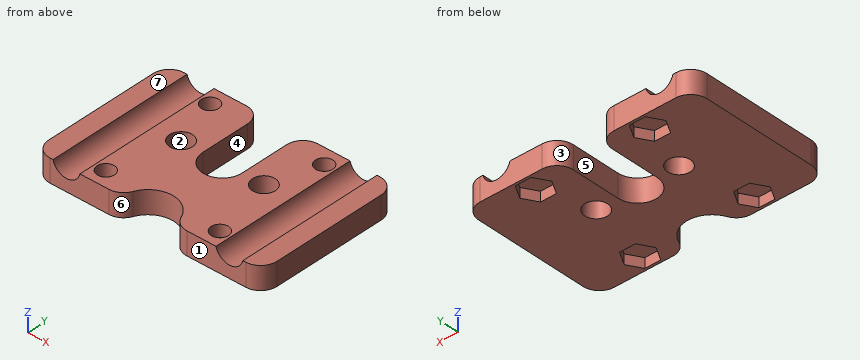
```python
from build123d import *

# Parameters (mm, degrees)
F0_R     = 3.5
F0_R_2   = 2.65
F1_DEPTH = 7
F2_DEPTH = 3
F3_R     = 4.25
F4_DEPTH = 45.001
F5_R     = 5
F7_R     = 2.65
F8_DEPTH = 0.25


with BuildPart() as f1:
    # F0 (on Top) → F1 (new body)
    with BuildSketch(Plane.XY):
        with BuildLine():
            Line((-6, 22.5), (-35, 22.5))
            Line((-35, 22.5), (-35, -22.5))
            Line((-35, -22.5), (-8, -22.5))
            ThreePointArc((-8, -22.5), (0, -14.5), (8, -22.5))
            Line((8, -22.5), (35, -22.5))
            Line((35, -22.5), (35, 22.5))
            Line((35, 22.5), (6, 22.5))
            Line((6, 22.5), (6, 2.5))
            ThreePointArc((6, 2.5), (0, -3.5), (-6, 2.5))
            Line((-6, 2.5), (-6, 22.5))
        make_face()
        Polygon((-22.4074772881, -17.5), (-19.9537386441, -13.25), (-15.0462613559, -13.25), (-12.5925227119, -17.5), (-15.0462613559, -21.75), (-19.9537386441, -21.75), align=None, mode=Mode.SUBTRACT)
        Polygon((12.5925227119, -17.5), (15.0462613559, -13.25), (19.9537386441, -13.25), (22.4074772881, -17.5), (19.9537386441, -21.75), (15.0462613559, -21.75), align=None, mode=Mode.SUBTRACT)
        with Locations((-12.7, 2.5)):
            Circle(F0_R, mode=Mode.SUBTRACT)
        Polygon((-12.5925227119, 17.5), (-15.0462613559, 13.25), (-19.9537386441, 13.25), (-22.4074772881, 17.5), (-19.9537386441, 21.75), (-15.0462613559, 21.75), align=None, mode=Mode.SUBTRACT)
        with Locations((12.7, 2.5)):
            Circle(F0_R, mode=Mode.SUBTRACT)
        Polygon((22.4074772881, 17.5), (19.9537386441, 13.25), (15.0462613559, 13.25), (12.5925227119, 17.5), (15.0462613559, 21.75), (19.9537386441, 21.75), align=None, mode=Mode.SUBTRACT)
        Polygon((-19.9537386441, 13.25), (-15.0462613559, 13.25), (-12.5925227119, 17.5), (-15.0462613559, 21.75), (-19.9537386441, 21.75), (-22.4074772881, 17.5), align=None)
        with Locations((-17.5, 17.5)):
            Circle(F0_R_2, mode=Mode.SUBTRACT)
        Polygon((-15.0462613559, -13.25), (-19.9537386441, -13.25), (-22.4074772881, -17.5), (-19.9537386441, -21.75), (-15.0462613559, -21.75), (-12.5925227119, -17.5), align=None)
        with Locations((-17.5, -17.5)):
            Circle(F0_R_2, mode=Mode.SUBTRACT)
        Polygon((19.9537386441, -13.25), (15.0462613559, -13.25), (12.5925227119, -17.5), (15.0462613559, -21.75), (19.9537386441, -21.75), (22.4074772881, -17.5), align=None)
        with Locations((17.5, -17.5)):
            Circle(F0_R_2, mode=Mode.SUBTRACT)
        Polygon((15.0462613559, 13.25), (19.9537386441, 13.25), (22.4074772881, 17.5), (19.9537386441, 21.75), (15.0462613559, 21.75), (12.5925227119, 17.5), align=None)
        with Locations((17.5, 17.5)):
            Circle(F0_R_2, mode=Mode.SUBTRACT)
    extrude(amount=F1_DEPTH)

    # F0 (on Top) → F2 (cut)
    with BuildSketch(Plane.XY):
        Polygon((19.9537386441, -13.25), (15.0462613559, -13.25), (12.5925227119, -17.5), (15.0462613559, -21.75), (19.9537386441, -21.75), (22.4074772881, -17.5), align=None)
        with Locations((17.5, -17.5)):
            Circle(F0_R_2, mode=Mode.SUBTRACT)
        Polygon((15.0462613559, 13.25), (19.9537386441, 13.25), (22.4074772881, 17.5), (19.9537386441, 21.75), (15.0462613559, 21.75), (12.5925227119, 17.5), align=None)
        with Locations((17.5, 17.5)):
            Circle(F0_R_2, mode=Mode.SUBTRACT)
        Polygon((-19.9537386441, 13.25), (-15.0462613559, 13.25), (-12.5925227119, 17.5), (-15.0462613559, 21.75), (-19.9537386441, 21.75), (-22.4074772881, 17.5), align=None)
        with Locations((-17.5, 17.5)):
            Circle(F0_R_2, mode=Mode.SUBTRACT)
        Polygon((-15.0462613559, -13.25), (-19.9537386441, -13.25), (-22.4074772881, -17.5), (-19.9537386441, -21.75), (-15.0462613559, -21.75), (-12.5925227119, -17.5), align=None)
        with Locations((-17.5, -17.5)):
            Circle(F0_R_2, mode=Mode.SUBTRACT)
    extrude(amount=F2_DEPTH, mode=Mode.SUBTRACT)

    # F3 (on face) → F4 (cut, through all)
    with BuildSketch(Plane(origin=(0, 22.5, 0), x_dir=(-1, 0, 0), z_dir=(0, 1, 0))):
        with Locations((-25, 8)):
            Circle(F3_R)
        with Locations((25, 8)):
            Circle(F3_R)
    extrude(amount=-F4_DEPTH, mode=Mode.SUBTRACT)

    # F5
    f5_edges = [f1.edges().sort_by_distance(p)[0] for p in [
        (35, 22.5, 3.5),
        (6, 22.5, 3.5),
        (-6, 22.5, 3.5),
        (-35, 22.5, 3.5),
        (-35, -22.5, 3.5),
        (35, -22.5, 3.5),
        (-8, -22.5, 3.5),
        (8, -22.5, 3.5),
    ]]
    fillet(f5_edges, radius=F5_R)

    # F7 (on offset) → F8 (join)
    with BuildSketch(Plane(origin=(0, 0, 3), x_dir=(1, 0, 0), z_dir=(0, 0, -1))):
        with Locations((17.5, -17.5)):
            Circle(F7_R)
        with Locations((17.5, 17.5)):
            Circle(F7_R)
        with Locations((-17.5, 17.5)):
            Circle(F7_R)
        with Locations((-17.5, -17.5)):
            Circle(F7_R)
    extrude(amount=-F8_DEPTH)


solid = f1.part
```
Here's how the part is built. I have some questions about the finished solid (model axes, mm). Face numbers are marked on the shaded views. A direction names the side the tool comes from. Coordinates: 2 decimals unless noted, no trailing zeros. Order: outer loops, then holes, each group sorted by start corner. A loop starts at its lowest first (then second) coordinate and runs counter-clockwise, first axis right, second up. Notation, with made-up numbers: (-16.75, -31.5) - (3.25, -31.5) arc R14 ccw to (3.25, -7.5) - close; hole circle Ø1 at (21, -28). An arc over 180 degrees is marked (long way). One line per question, with ' | ' between items. Start each with the question number.
1. If we section it at A-A (y = -16): Write out the boundary of the cut face in (x, z).
2. If we section it at D-D (y = -5): Write out the boundary of the cut face in (x, z), and give its area (3 significant figures).
3. If we section it at B-B (x = -13.5): Write out the boundary of the cut face in (y, z), and give its area (3 significant figures).
4. Which directions (+Z, -Z, +X, -X, +Y, -Y) give clear straight access to the entire face, cutting with the end or side of a thin tool? Please do the marked faces 5, 6 and 7.
5. If we mould it in two halves opening along Y, with no side actions, what happens to the marked faces 1, 2, 3 and 4? For each: released by +Y, released by -Y, zero draft, split by the parting line, or undercut.
6. I'm going to push flat-ended pins straight in: pin 1 Ø1.6 at (x, y) = (16.5, 17) entering from +Z; pin 2 Ø2.5 at (x, y) = (-17, -16) entering from -Z. Where does each tip first touch, or does it pass through?
7. Please list where these lines run through material, in increasing order: line 1 along Y through (x, z) = (17.5, 4); line 2 along Y through (x, z) = (19, 1.5); line 3 along X through (y, z) = (4.5, 4.5). Write a range as [from, to].
8. If we section it at C-C (z = 6.25): Give the number of separate pieces and of enclosed holes in the cut face, and give its area (3 significant figures).
Model answer:
1) outline: (-35, 0) - (-21.54, 0) - (-21.54, 3) - (-13.46, 3) - (-13.46, 0) - (-4.66, 0) - (-4.66, 7) - (-15.32, 7) - (-15.32, 3.25) - (-19.68, 3.25) - (-19.68, 7) - (-20.87, 7) arc R4.25 cw to (-29.13, 7) - (-35, 7) - close; (4.66, 0) - (13.46, 0) - (13.46, 3) - (21.54, 3) - (21.54, 0) - (35, 0) - (35, 7) - (29.13, 7) arc R4.25 cw to (20.87, 7) - (19.68, 7) - (19.68, 3.25) - (15.32, 3.25) - (15.32, 7) - (4.66, 7) - close
2) outline: (-35, 0) - (35, 0) - (35, 7) - (29.13, 7) arc R4.25 cw to (20.87, 7) - (-20.87, 7) arc R4.25 cw to (-29.13, 7) - (-35, 7) - close | area: 450 mm²
3) outline: (-22.5, 0) - (-19.07, 0) - (-19.07, 3) - (-15.93, 3) - (-15.93, 0) - (-0.91, 0) - (-0.91, 7) - (-22.5, 7) - close; (5.91, 0) - (15.93, 0) - (15.93, 3) - (19.07, 3) - (19.07, 0) - (22.5, 0) - (22.5, 7) - (5.91, 7) - close | area: 248 mm²
4) face 5: +Z, -Z, +Y | face 6: +Z, -Z, -Y | face 7: +Z, +X, -X, +Y, -Y
5) face 1: released by -Y | face 2: undercut | face 3: released by +Y | face 4: zero draft
6) pin 1: stops at z = 3.25 | pin 2: stops at z = 3
7) line 1: y = [-22.5, -20.15], [-14.85, 14.85], [20.15, 22.5] | line 2: y = [-22.5, -21.75], [-13.25, 13.25], [21.75, 22.5] | line 3: x = [-35, -27.41], [-22.59, -15.57], [-9.83, -6], [6, 9.83], [15.57, 22.59], [27.41, 35]
8) separate pieces: 3 | enclosed holes: 6 | area: 1,850 mm²
